Input: part model. Units: mm. Frame: model coordinates. A direction names the side the tool comes from. Give positions to 0.01 mm unless a question says otherwise; leave off trailing zeros. Loops run counter-clockwise (first coordinate to the right, second up) from the corner with the lowest first, then second, coordinate; pieces in that order, holes last.
from build123d import *

# Parameters (mm, degrees)
BOSS_EXTRUDE1_DEPTH            = 32
CBORE_FOR_M8_SHCS1_D           = 10
CBORE_FOR_M8_SHCS1_CBORE_D     = 14
CBORE_FOR_M8_SHCS1_CBORE_DEPTH = 8


with BuildPart() as part:
    # Sketch1 → Boss-Extrude1 (new body)
    with BuildSketch(Plane.XY):
        with BuildLine():
            Line((-13, 0), (-30, 0))
            Line((-30, 0), (-30, 20))
            Line((-30, 20), (30, 20))
            Line((30, 20), (30, 0))
            Line((30, 0), (13, 0))
            ThreePointArc((13, 0), (0, 13), (-13, 0))
        make_face()
    extrude(amount=BOSS_EXTRUDE1_DEPTH)

    # CBORE for M8 SHCS1 (through all)
    with Locations(Plane(origin=(0, 20, 0), x_dir=(1, 0, 0), z_dir=(0, 1, 0))):
        with Locations((-19, -16), (19, -16)):
            CounterBoreHole(CBORE_FOR_M8_SHCS1_D / 2, CBORE_FOR_M8_SHCS1_CBORE_D / 2, CBORE_FOR_M8_SHCS1_CBORE_DEPTH)


solid = part.part
(1) Cut plane D-D (z = 8). Return the cut outline in (x, y), and give its area (3 significant figures).
Values follow:
outline: (-30, 0) - (-13, 0) arc R13 cw to (13, 0) - (30, 0) - (30, 20) - (-30, 20) - close
area: 935 mm2
(2) Cut plane C-C (z = 16). Return the cut outline in (x, y).
Values follow:
outline: (-30, 0) - (-24, 0) - (-24, 12) - (-26, 12) - (-26, 20) - (-30, 20) - close; (-14, 0) - (-13, 0) arc R13 cw to (13, 0) - (14, 0) - (14, 12) - (12, 12) - (12, 20) - (-12, 20) - (-12, 12) - (-14, 12) - close; (24, 0) - (30, 0) - (30, 20) - (26, 20) - (26, 12) - (24, 12) - close
(3) Cut plane B-B (x = -19). Return the cut outline in (y, z), and give its area (3 significant figures).
Values follow:
outline: (0, 0) - (20, 0) - (20, 9) - (12, 9) - (12, 11) - (0, 11) - close; (0, 21) - (12, 21) - (12, 23) - (20, 23) - (20, 32) - (0, 32) - close
area: 408 mm2
(4) Mould query, pull axis X, two halves, no side actions, for faces 3 (the flat face through (0, 15, 32)), 4 (the cylindrical face through (20.08, 5.92, 20.88)), 5 (the flat face through (30, 10, 16)). Classes: +X half, -X half, draft (parallel to the pull), parting line (faces both ways), or undercut.
Values follow:
face 3: draft
face 4: undercut
face 5: +X half
(5) Ray query, probe 1 along X at (y, z) = (15.5, 16); probe 2 along Z at (x, y) = (-19, 7); probe 3 along X at (y, z) = (17.25, 17). Return the intervals inside material, ascending.
Values follow:
probe 1: x = -30 to -26, -12 to 12, 26 to 30
probe 2: z = 0 to 11, 21 to 32
probe 3: x = -30 to -25.93, -12.07 to 12.07, 25.93 to 30
(6) Reachability of faces 1 (the flat face through (-30, 10, 16)), 2 (the cylindrical face through (12, 16, 16)) from +Z, -Z, +X, -X, +Y, -Y: full face, straight path, thin tool, end or side. Return the list, or none.
Values follow:
face 1: +Z, -Z, -X, +Y, -Y
face 2: +Y
(7) Cut plane A-A (y = 7). Return the cut outline in (x, z), and give its area (3 significant figures).
Values follow:
outline: (-30, 0) - (-10.95, 0) - (-10.95, 32) - (-30, 32) - close; (10.95, 0) - (30, 0) - (30, 32) - (10.95, 32) - close; hole circle Ø10 at (-19, 16); hole circle Ø10 at (19, 16)
area: 1,060 mm2
